Source: CAD feature listing. Evaluate the final solid. Frame: model axes, mm. A direction names the side the tool comes from. Give positions to 0.01 mm unless a question says otherwise; leave off trailing zeros. Order: outer loops, then holes, each group sorted by start corner. A loop starts at its lowest first (then second) coordinate and runs counter-clockwise, first axis right, second up.
```python
from build123d import *

# Parameters (mm, degrees)
SKETCH_1_W             = 19
SKETCH_1_H             = 30
SKETCH_1_R             = 1.5
SM_BASE_FLANGE_1_DEPTH = 1
FILLET_1_R             = 2


# Sheet-metal steps are written as plain solids
with BuildPart() as part:
    # Sketch 1 → 基体-法兰1 (new body)
    with BuildSketch(Plane(origin=(0, 0, 0), x_dir=(1, 0, 0), z_dir=(0, 1, 0))):
        with Locations((0, 11.5)):
            Rectangle(SKETCH_1_W, SKETCH_1_H)
        with Locations(Location((-6.4, 0, 0), (0, 0, 270))):
            Circle(SKETCH_1_R, mode=Mode.SUBTRACT)
        with Locations(Location((6.4, 0, 0), (0, 0, 270))):
            Circle(SKETCH_1_R, mode=Mode.SUBTRACT)
        with BuildLine():
            Line((-2.5, 22), (-2.5, 20))
            ThreePointArc((-2.5, 20), (-4, 18.5), (-5.5, 20))
            Line((-5.5, 20), (-5.5, 22))
            ThreePointArc((-5.5, 22), (-4, 23.5), (-2.5, 22))
        make_face(mode=Mode.SUBTRACT)
        with BuildLine():
            Line((5.5, 22), (5.5, 20))
            ThreePointArc((5.5, 20), (4, 18.5), (2.5, 20))
            Line((2.5, 20), (2.5, 22))
            ThreePointArc((2.5, 22), (4, 23.5), (5.5, 22))
        make_face(mode=Mode.SUBTRACT)
    extrude(amount=-SM_BASE_FLANGE_1_DEPTH)

    # 圆角1
    fillet_1_edges = [part.edges().sort_by_distance(p)[0] for p in [
        (9.5, -0.5, -26.5),
        (9.5, -0.5, 3.5),
        (-9.5, -0.5, 3.5),
        (-9.5, -0.5, -26.5),
    ]]
    fillet(fillet_1_edges, radius=FILLET_1_R)


solid = part.part
```
1) Section query D-D, the plane x = 4. Return the cut outline in (y, z).
Report:
outline: (-1, -26.5) - (0, -26.5) - (0, -23.5) - (-1, -23.5) - close; (-1, -18.5) - (0, -18.5) - (0, 3.5) - (-1, 3.5) - close
2) Section query C-C, the plane y = -0.5. Return the cut outline in (x, z).
Report:
outline: (-9.5, -24.5) arc R2 ccw to (-7.5, -26.5) - (7.5, -26.5) arc R2 ccw to (9.5, -24.5) - (9.5, 1.5) arc R2 ccw to (7.5, 3.5) - (-7.5, 3.5) arc R2 ccw to (-9.5, 1.5) - close; hole circle Ø3 at (-6.4, 0); hole (-5.5, -22) arc R1.5 ccw to (-2.5, -22) - (-2.5, -20) arc R1.5 ccw to (-5.5, -20) - close; hole (2.5, -22) arc R1.5 ccw to (5.5, -22) - (5.5, -20) arc R1.5 ccw to (2.5, -20) - close; hole circle Ø3 at (6.4, 0)
3) Draft query along Z for faces 1 (the cylindrical face through (-5.95, -0.49, 1.43)), 2 (the flat face through (-0.1, -0.5, -26.5)), 3 (the flat face through (-9.5, -0.5, -11.3)), 4 (the cylindrical face through (-8.93, -0.51, 2.9)). Return one class per face: +Z half, -Z half, draft (parallel to the pull), parting line (faces both ways), or undercut.
Report:
face 1: undercut
face 2: -Z half
face 3: draft
face 4: +Z half
4) Material intervals for L1, parallel to X at y = -0.25, z = 0; L2, parallel to X at y = -0.55, z = -0.75; L3, parallel to Z at x = 7.75, y = -0.7, sorted ascending.
Report:
L1: x = -9.5 to -7.9, -4.9 to 4.9, 7.9 to 9.5
L2: x = -9.5 to -7.7, -5.1 to 5.1, 7.7 to 9.5
L3: z = -26.48 to -0.65, 0.65 to 3.48
5) Reachability of faces 5 (the flat face through (0, -1, -12)), 6 (the cylindrical face through (-4, -0.5, -18.5)) from +Z, -Z, +X, -X, +Y, -Y: full face, straight path, thin tool, end or side. Return the list, or none.
Report:
face 5: +Z, -Z, +X, -X, -Y
face 6: +Y, -Y
6) Section query B-B, the plane z = 0. Return the cut outline in (x, y), and give its area (3 significant figures).
Report:
outline: (-9.5, -1) - (-7.9, -1) - (-7.9, 0) - (-9.5, 0) - close; (-4.9, -1) - (4.9, -1) - (4.9, 0) - (-4.9, 0) - close; (7.9, -1) - (9.5, -1) - (9.5, 0) - (7.9, 0) - close
area: 13.0 mm2
7) Section query A-A, the plane x = -6.4. Return the cut outline in (y, z), and give its area (3 significant figures).
Report:
outline: (-1, -26.5) - (0, -26.5) - (0, -1.5) - (-1, -1.5) - close; (-1, 1.5) - (0, 1.5) - (0, 3.5) - (-1, 3.5) - close
area: 27.0 mm2
